The model under review builds one solid part; all positions refer to its coordinate system, in mm. Face numbers are marked on the shaded views. Give positions to 0.01 mm unless a question says otherwise; leave off trailing zeros. Order: outer loops, then holes, each group sorted by start corner. A loop starts at its lowest first (then second) coordinate and runs counter-clockwise, first axis right, second up. Notation, with made-up numbers: M 51,11 L 86,11 A7 ccw 86,19 Z; hole C 71,37.25 d8. An arc over 180 degrees is marked long. One line per question, with ' | ' between items. Start each with the question number.
1. We need section A-A on x = -49.5. Write out the cut boundary in (y, z), then the cut area to 3 significant figures.
2. Wall thickness on L1, parallel to Z at x = -36, y = 77; L2, parallel to Z at x = 96.5, y = 80; L3, parallel to Y at x = -38, z = -9: over which ranges is each line inside the solid? List them lowest first.
3. The part is to be moulded in two halves that separate along X. For the marked faces 1, 2, 3 and 4, say which applies: +X half, -X half, draft (parallel to the pull), parting line (faces both ways), or undercut.
4. Insertion check: P1, Ø16, axis at x = -105.38, z = 50.47, coming from the +Y side; P2, Ø12, axis at x = 105.38, z = 50.47, coming from the +Y side. Each pin has a flat end and moves straight along its axis. Give the tip position at first contact, or say it passes through.
5. We need section B-B on z = -5.5. Write out the cut boundary in (x, y).
```python
from build123d import *

# Parameters (mm, degrees)
SKETCH3_W                  = 240.765342714
SKETCH3_H                  = 130.947670476
BOSS_EXTRUDE2_DEPTH        = 85
SKETCH4_W                  = 180.765342714
SKETCH4_H                  = 70.947670476
CUT_EXTRUDE1_DEPTH         = 15
F_20_0MM_DOWEL_HOLE1_D     = 20
F_20_0MM_DOWEL_HOLE1_DEPTH = 10.05
F_20_0MM_DOWEL_HOLE1_TIP   = 6.00860619
FILLET1_R                  = 20


with BuildPart() as part:
    # Sketch3 → Boss-Extrude2 (new body)
    with BuildSketch(Plane(origin=(0, 0, 0), x_dir=(1, 0, 0), z_dir=(0, 1, 0))):
        Rectangle(SKETCH3_W, SKETCH3_H)
    extrude(amount=BOSS_EXTRUDE2_DEPTH)

    # Sketch4 → Cut-Extrude1 (cut)
    with BuildSketch(Plane(origin=(0, 85, 0), x_dir=(1, 0, 0), z_dir=(0, 1, 0))):
        Rectangle(SKETCH4_W, SKETCH4_H)
    extrude(amount=-CUT_EXTRUDE1_DEPTH, mode=Mode.SUBTRACT)

    # Ø20.0mm Dowel Hole1
    with Locations(Plane(origin=(-105.382671357, 85, -50.473835238), x_dir=(0, 0, 1), z_dir=(0, 1, 0))):
        with Locations((0, 0), (100.947670476, 0), (0, 210.765342714), (100.947670476, 210.765342714)):
            Hole(F_20_0MM_DOWEL_HOLE1_D / 2, depth=F_20_0MM_DOWEL_HOLE1_DEPTH)
            with Locations((0, 0, -(F_20_0MM_DOWEL_HOLE1_DEPTH + F_20_0MM_DOWEL_HOLE1_TIP / 2))):  # 118° drill point
                Cone(0, F_20_0MM_DOWEL_HOLE1_D / 2, F_20_0MM_DOWEL_HOLE1_TIP, mode=Mode.SUBTRACT)

    # Fillet1
    fillet1_edges = [part.edges().sort_by_distance(p)[0] for p in [
        (90.382671357, 77.5, 35.473835238),
        (-90.382671357, 77.5, 35.473835238),
        (-90.382671357, 77.5, -35.473835238),
        (90.382671357, 77.5, -35.473835238),
    ]]
    fillet(fillet1_edges, radius=FILLET1_R)


solid = part.part
```
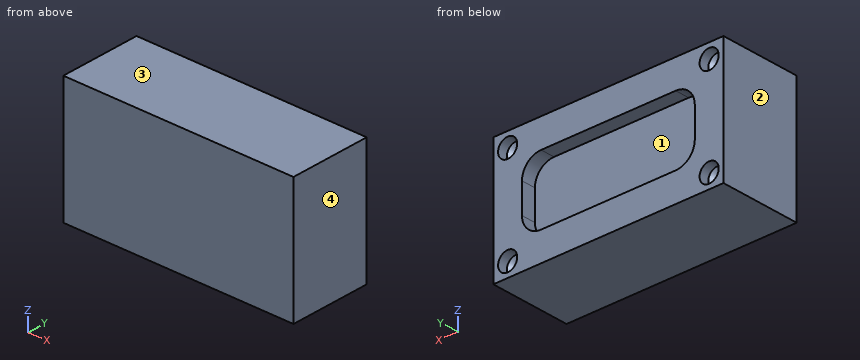
Entries:
1) outline: M 0,-65.47 L 85,-65.47 L 85,-35.47 L 70,-35.47 L 70,35.47 L 85,35.47 L 85,65.47 L 0,65.47 Z | area: 10,100 mm^2
2) L1: z = -65.47 to -35.47, 35.47 to 65.47 | L2: z = -65.47 to -55.07, -45.88 to 45.88, 55.07 to 65.47 | L3: y = 0 to 70
3) face 1: undercut | face 2: -X half | face 3: draft | face 4: +X half
4) P1: stops at y = 73.75 | P2: stops at y = 72.55
5) outline: M -120.38,0 L 120.38,0 L 120.38,85 L 90.38,85 L 90.38,70 L -90.38,70 L -90.38,85 L -120.38,85 Z
